CAD build for the part. Positions are in the model's coordinates, mm. Round coordinates to 2 decimals unless told otherwise and drop trailing zeros. Order: outer loops, then holes, each group sorted by start corner. A loop starts at its lowest first (then second) coordinate and runs counter-clockwise, first axis right, second up.
```python
from build123d import *

# Parameters (mm, degrees)
SKETCH048_R            = 3.571875
PAD048_DEPTH           = 13
SKETCH047_R            = 34.925
SKETCH047_R_2          = 9.525
PAD047_DEPTH           = 12.7
CUT041_PLACEMENT_ANGLE = 60
CUT042_PLACEMENT_ANGLE = 60
CUT043_PLACEMENT_ANGLE = 60
CUT044_PLACEMENT_ANGLE = 60
CUT045_PLACEMENT_ANGLE = 60
CHAMFER005_SIZE        = 1.59
CHAMFER004_SIZE        = 0.79


with BuildPart() as body049:
    # Sketch048 → Pad048 (new body)
    with BuildSketch(Plane.XZ):
        with Locations((0, 29.36875)):
            Circle(SKETCH048_R)
    extrude(amount=PAD048_DEPTH)


with BuildPart() as chamfer004:
    # Sketch047 → Pad047 (new body)
    with BuildSketch(Plane.XZ):
        Circle(SKETCH047_R)
        Circle(SKETCH047_R_2, mode=Mode.SUBTRACT)
    extrude(amount=PAD047_DEPTH)

    # Cut041: cut Body049
    add(body049.part, mode=Mode.SUBTRACT)


with BuildPart() as chamfer004_1:
    # Cut041 placement: moved
    add(chamfer004.part.rotate(Axis((0, 0, 0), (0, 1, 0)), CUT041_PLACEMENT_ANGLE))

    # Cut042: cut Body049
    add(body049.part, mode=Mode.SUBTRACT)


with BuildPart() as chamfer004_2:
    # Cut042 placement: moved
    add(chamfer004_1.part.rotate(Axis((0, 0, 0), (0, 1, 0)), CUT042_PLACEMENT_ANGLE))

    # Cut043: cut Body049
    add(body049.part, mode=Mode.SUBTRACT)


with BuildPart() as chamfer004_3:
    # Cut043 placement: moved
    add(chamfer004_2.part.rotate(Axis((0, 0, 0), (0, 1, 0)), CUT043_PLACEMENT_ANGLE))

    # Cut044: cut Body049
    add(body049.part, mode=Mode.SUBTRACT)


with BuildPart() as chamfer004_4:
    # Cut044 placement: moved
    add(chamfer004_3.part.rotate(Axis((0, 0, 0), (0, 1, 0)), CUT044_PLACEMENT_ANGLE))

    # Cut045: cut Body049
    add(body049.part, mode=Mode.SUBTRACT)


with BuildPart() as chamfer004_5:
    # Cut045 placement: moved
    add(chamfer004_4.part.rotate(Axis((0, 0, 0), (0, 1, 0)), CUT045_PLACEMENT_ANGLE))

    # Cut046: cut Body049
    add(body049.part, mode=Mode.SUBTRACT)

    # Chamfer005
    chamfer005_edges = [chamfer004_5.edges().sort_by_distance(p)[0] for p in [
        (-17.4625, -12.7, -30.245937),
    ]]
    chamfer(chamfer005_edges, length=CHAMFER005_SIZE)

    # Chamfer004
    chamfer004_edges = [chamfer004_5.edges().sort_by_distance(p)[0] for p in [
        (-17.4625, 0, -30.245937),
    ]]
    chamfer(chamfer004_edges, length=CHAMFER004_SIZE)


solid = chamfer004_5.part
```
1. Cut at A-A, the plane x = 0. Write the cut outline in (y, z) (3 decimals).
2. Cut at C-C, the plane y = -8.5. Give the number of separate pieces and of enclosed holes in the cut face, and give its area (3 significant figures).
3. Cut at B-B, the plane z = 0. Write the cut outline in (x, y) (3 decimals), and give its area (3 significant figures).
4. Pin check, flat tips, straight feed: P1, Ø4, axis at x = -13, y = -8, coming from the -Z side; P2, Ø2, axis at x = 4, y = -6, coming from the +Z side; P3, Ø6.5, axis at x = 0, z = -29.37, coming from the -Y side; P4, Ø2, axis at y = -8, z = -24.5, coming from the +X side. Stop position of each tip, or through.
5. Drill centre lines: line 1 (X direction, y = -9.25, z = -16.5); line 2 (Z direction, x = -23.5, y = -4.25); line 3 (Z direction, x = -0.5, y = -1.75). Where is each one in solid material? Low to high.
6. Mould opens along Z. For faces 1 (the face through (7.571, -5.878, 34.094)), 2 (the face through (7.02, -6.26, -6.44)), 3 (the face through (10, 0, 3)) say: released by +Z, released by -Z, zero draft, split by the parting line, or undercut.
Outcome:
1. outline: (-12.7, -33.335) - (-11.11, -34.925) - (-0.79, -34.925) - (0, -34.135) - (0, -32.941) - (-12.7, -32.941) - close; (-12.7, -25.797) - (0, -25.797) - (0, -9.525) - (-12.7, -9.525) - close; (-12.7, 9.525) - (0, 9.525) - (0, 25.797) - (-12.7, 25.797) - close; (-12.7, 32.941) - (0, 32.941) - (0, 34.135) - (-0.79, 34.925) - (-11.11, 34.925) - (-12.7, 33.335) - close
2. separate pieces: 1
2. enclosed holes: 7
2. area: 3,310 mm2
3. outline: (-34.925, -11.11) - (-33.335, -12.7) - (-9.525, -12.7) - (-9.525, 0) - (-34.135, 0) - (-34.925, -0.79) - close; (9.525, -12.7) - (33.335, -12.7) - (34.925, -11.11) - (34.925, -0.79) - (34.135, 0) - (9.525, 0) - close
3. area: 642 mm2
4. P1: stops at z = -33.15
4. P2: stops at z = 34.8
4. P3: passes through
4. P4: stops at x = 25.84
5. line 1: x = -30.78 to -28.51, -22.36 to 22.36, 28.51 to 30.78
5. line 2: z = -25.84 to -17.69, -11.68 to 11.68, 17.69 to 25.84
5. line 3: z = -34.92 to -32.91, -25.83 to -9.51, 9.51 to 25.83, 32.91 to 34.92
6. face 1: split by the parting line
6. face 2: undercut
6. face 3: zero draft
